CAD build for the part. Positions are in the model's coordinates, mm. Round coordinates to 2 decimals unless told otherwise and drop trailing zeros. Write each loop counter-clockwise with the first axis right and the second up, starting at its lowest first coordinate (ties: lowest second). Pieces come first, ordered by that corner, then holes. Notation, with made-up numbers: (28, 5.25) - (82, 5.25) arc R21 ccw to (82, 24.25) - close; hole circle Ø11 at (26, 4.25). An arc over 180 degrees is marked (long way). Put each result on its own line as item: value. Start each with the question number.
Item 1: Cut at B-B (y = 2). Count the separate pieces of the cut face and the enclosed holes in it, and give its area (3 significant figures).
Item 2: Mould opens along Z. For faces 1 (the flat face through (84, 3, -10)), 2 (the cylindrical face through (111.5, 1.52, -5.23)), 3 (the flat face through (84, 1, -20)) say: released by +Z, released by -Z, zero draft, split by the parting line, or undercut.
Item 3: Cut at A-A (x = 110). Give the cut face in (y, z), and give its area (3 significant figures).
Item 4: Drill centre lines: line 1 (X direction, y = 1.85, z = -10); line 2 (Z direction, x = 109.5, y = 1.7); line 3 (X direction, y = 2.8, z = -5.5). Where is each one in solid material? Low to high. Write a range as from..to.
Item 5: Cut at C-C (z = -16.75). Give the cut face in (x, y), and give its area (3 significant figures).
```python
from build123d import *

# Parameters (mm, degrees)
SKETCH2_W           = 170
SKETCH2_H           = 20
BOSS_EXTRUDE1_DEPTH = 3
SKETCH3_R           = 5
CUT_EXTRUDE1_DEPTH  = 172.198714948
SKETCH4_R           = 5
CUT_EXTRUDE2_DEPTH  = 172.198714948
FILLET1_R           = 10
FILLET2_R           = 10
SKETCH5_R           = 5
CUT_EXTRUDE3_DEPTH  = 172.198714948


with BuildPart() as part:
    # Sketch2 → Boss-Extrude1 (new body)
    with BuildSketch(Plane(origin=(0, 0, 0), x_dir=(1, 0, 0), z_dir=(0, 1, 0))):
        with Locations((85, 10)):
            Rectangle(SKETCH2_W, SKETCH2_H)
    extrude(amount=BOSS_EXTRUDE1_DEPTH)

    # Sketch3 → Cut-Extrude1 (cut, through all)
    with BuildSketch(Plane(origin=(0, 3, 0), x_dir=(1, 0, 0), z_dir=(0, 1, 0))):
        with Locations(Location((9, 10, 0), (0, 0, 270))):
            Circle(SKETCH3_R)
    extrude(amount=-CUT_EXTRUDE1_DEPTH, mode=Mode.SUBTRACT)

    # Sketch4 → Cut-Extrude2 (cut, through all)
    with BuildSketch(Plane(origin=(0, 3, 0), x_dir=(1, 0, 0), z_dir=(0, 1, 0))):
        with Locations(Location((161, 10, 0), (0, 0, 270))):
            Circle(SKETCH4_R)
    extrude(amount=-CUT_EXTRUDE2_DEPTH, mode=Mode.SUBTRACT)

    # Fillet1
    fillet1_edges = [part.edges().sort_by_distance(p)[0] for p in [
        (0, 1.5, -20),
        (0, 1.5, 0),
    ]]
    fillet(fillet1_edges, radius=FILLET1_R - 0.0001)  # a hair under: the kernel refuses the full size

    # Fillet2
    fillet2_edges = [part.edges().sort_by_distance(p)[0] for p in [
        (170, 1.5, -20),
        (170, 1.5, 0),
    ]]
    fillet(fillet2_edges, radius=FILLET2_R - 0.0001)  # a hair under: the kernel refuses the full size

    # Sketch5 → Cut-Extrude3 (cut, through all)
    with BuildSketch(Plane(origin=(0, 3, 0), x_dir=(1, 0, 0), z_dir=(0, 1, 0))):
        with Locations(Location((110, 10, 0), (0, 0, 270))):
            Circle(SKETCH5_R)
    extrude(amount=-CUT_EXTRUDE3_DEPTH, mode=Mode.SUBTRACT)


solid = part.part
```
Output values:
1. separate pieces: 1
1. enclosed holes: 3
1. area: 3,080 mm2
2. face 1: zero draft
2. face 2: undercut
2. face 3: released by -Z
3. outline: (0, -20) - (3, -20) - (3, -15) - (0, -15) - close; (0, -5) - (3, -5) - (3, 0) - (0, 0) - close
3. area: 30.0 mm2
4. line 1: 0..4, 14..105, 115..156, 166..170
4. line 2: -20..-14.97, -5.03..0
4. line 3: 1.07..6.82, 11.18..107.82, 112.18..158.82, 163.18..168.93
5. outline: (2.62, 0) - (167.38, 0) - (167.38, 3) - (2.62, 3) - close
5. area: 494 mm2
